```python
from build123d import *

# Parameters (mm, degrees)
BOSS_EXTRUDE1_DEPTH = 12
CUT_EXTRUDE1_DEPTH  = 22.9544984
SKETCH3_R           = 2
CUT_EXTRUDE2_DEPTH  = 22.9544984
FILLET1_R           = 6


with BuildPart() as part:
    # Sketch1 → Boss-Extrude1 (new body)
    with BuildSketch(Plane.XY):
        Polygon((0, 0), (13, 0), (13, 1), (1, 1), (1, 13), (0, 13), align=None)
    extrude(amount=BOSS_EXTRUDE1_DEPTH)

    # Sketch2 → Cut-Extrude1 (cut, through all)
    with BuildSketch(Plane.ZY):
        with BuildLine():
            Line((4, 5.5), (4, 7.5))
            ThreePointArc((4, 7.5), (6, 9.5), (8, 7.5))
            Line((8, 7.5), (8, 5.5))
            ThreePointArc((8, 5.5), (6, 3.5), (4, 5.5))
        make_face()
    extrude(amount=-CUT_EXTRUDE1_DEPTH, mode=Mode.SUBTRACT)

    # Sketch3 → Cut-Extrude2 (cut, through all)
    with BuildSketch(Plane.XZ):
        with Locations(Location((6.5, 6, 0), (0, 0, 270))):
            Circle(SKETCH3_R)
    extrude(amount=-CUT_EXTRUDE2_DEPTH, mode=Mode.SUBTRACT)

    # Fillet1
    fillet1_edges = [part.edges().sort_by_distance(p)[0] for p in [
        (0.5, 13, 0),
        (13, 0.5, 0),
        (13, 0.5, 12),
        (0.5, 13, 12),
    ]]
    fillet(fillet1_edges, radius=FILLET1_R - 0.0001)  # a hair under: the kernel refuses the full size


solid = part.part
```
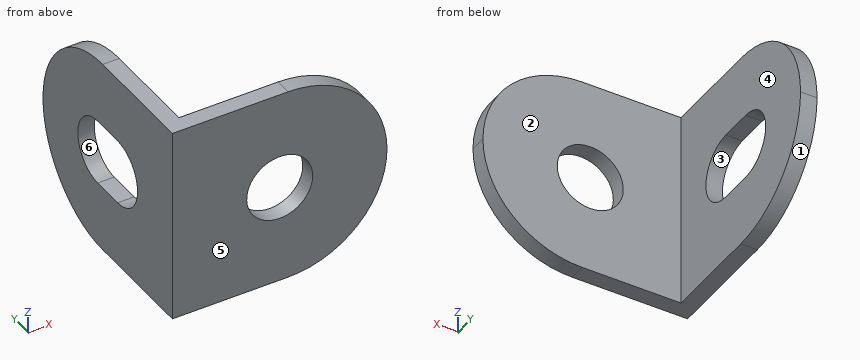
Build history of the part. All positions in model axes, mm. Face numbers are marked on the shaded views. A direction names the side the tool comes from. Round coordinates to 2 decimals unless told otherwise and drop trailing zeros. Order: outer loops, then holes, each group sorted by start corner. A loop starts at its lowest first (then second) coordinate and runs counter-clockwise, first axis right, second up. Notation, with made-up numbers: (45, 81) -> (83, 81) arc R30 ccw to (83, 107) -> close; hole circle Ø3 at (40.25, 15). An arc over 180 degrees is marked (long way). Answer in a Markdown table with one row per item.
1) Band-saw the part on B-B on z = 5.25. Give the cut face in (x, y).
Values:
| item | result |
|---|---|
| outline | (0, 0) -> (4.65, 0) -> (4.65, 1) -> (1, 1) -> (1, 3.65) -> (0, 3.65) -> close; (0, 9.35) -> (1, 9.35) -> (1, 12.95) -> (0, 12.95) -> close; (8.35, 0) -> (12.95, 0) -> (12.95, 1) -> (8.35, 1) -> close |
2) Band-saw the part on C-C on y = 9. Give the cut face in (x, z).
Values:
| item | result |
|---|---|
| outline | (0, 0.34) -> (1, 0.34) -> (1, 4.68) -> (0, 4.68) -> close; (0, 7.32) -> (1, 7.32) -> (1, 11.66) -> (0, 11.66) -> close |
3) Mould opens along Y. For the marked faces 3, 4, 5 and 6 say: released by +Y, released by -Y, zero draft, split by the parting line, or undercut.
Values:
| item | result |
|---|---|
| face 3 | undercut |
| face 4 | zero draft |
| face 5 | released by -Y |
| face 6 | undercut |
4) Wall check: L1, parallel to X at y = 0.55, z = 6; L2, parallel to X at y = 9.5, z = 3.75. Give the ranges that are in metal, low to high.
Values:
| item | result |
|---|---|
| L1 | 0 to 4.5, 8.5 to 13 |
| L2 | 0 to 1 |
5) Band-saw the part on D-D on z = 7.75. Give the cut face in (x, y).
Values:
| item | result |
|---|---|
| outline | (0, 0) -> (5.53, 0) -> (5.53, 1) -> (1, 1) -> (1, 4.53) -> (0, 4.53) -> close; (0, 8.47) -> (1, 8.47) -> (1, 12.74) -> (0, 12.74) -> close; (7.47, 0) -> (12.74, 0) -> (12.74, 1) -> (7.47, 1) -> close |
6) Band-saw the part on A-A on x = 7.75. Give the cut face in (y, z).
Values:
| item | result |
|---|---|
| outline | (0, 0.05) -> (1, 0.05) -> (1, 4.44) -> (0, 4.44) -> close; (0, 7.56) -> (1, 7.56) -> (1, 11.95) -> (0, 11.95) -> close |
7) Which spindle directions (+Z, -Z, +X, -X, +Y, -Y) get a long thin tool onto all of the face, cutting with end or side? Do the marked faces 1 and 2. Say none if no direction does.
Values:
| item | result |
|---|---|
| face 1 | -Z, +X, -X, +Y |
| face 2 | +Z, -Z, +X, +Y |
8) Pin check, flat tips, straight feed: P1, Ø4, axis at x = 1.5, y = 11, coming from the -Z side; P2, Ø3, axis at y = 10.5, z = 10, coming from the +X side. Stop position of each tip, or through.
Values:
| item | result |
|---|---|
| P1 | z = 0.37 |
| P2 | x = 1 |
